For this review, take the finished solid that the model builds, in its own axes (mm). A direction names the side the tool comes from. Give positions to 0.01 mm unless a question says otherwise; leave off trailing zeros. Loops run counter-clockwise (first coordinate to the right, second up) from the corner with the lowest first, then second, coordinate; pieces in that order, holes last.
Autodesk Inventor part; units mm, degrees
ref_plane "YZ Plane" through (0, 0, 0) normal (1, 0, 0) x (0, 1, 0)
ref_plane "XZ Plane" through (0, 0, 0) normal (0, 1, 0) x (-1, 0, 0)
ref_plane "XY Plane" through (0, 0, 0) normal (0, 0, 1) x (1, 0, 0)
sketch "Boceto1" plane through (0, 0, 0) normal (1, 0, 0) x (0, 1, 0)
  line L0 (0, 0) -> (19, 0)
  line L1 (19, 0) -> (19, -90)
  line L2 (19, -90) -> (0, -90)
  line L3 (0, -90) -> (0, 0)
  line L4 (19, -7.5) -> (22, -7.5)
  line L5 (22, -7.5) -> (22, -22.5)
  line L6 (22, -22.5) -> (19, -22.5)
  line L7 (19, -22.5) -> (19, -7.5)
  line L8 (19, -27.5) -> (22, -27.5)
  line L9 (22, -27.5) -> (22, -42.5)
  line L10 (22, -42.5) -> (19, -42.5)
  line L11 (19, -42.5) -> (19, -27.5)
  line L12 (19, -47.5) -> (22, -47.5)
  line L13 (22, -47.5) -> (22, -62.5)
  line L14 (22, -62.5) -> (19, -62.5)
  line L15 (19, -62.5) -> (19, -47.5)
  line L16 (19, -67.5) -> (22, -67.5)
  line L17 (22, -67.5) -> (22, -82.5)
  line L18 (22, -82.5) -> (19, -82.5)
  line L19 (19, -82.5) -> (19, -67.5)
  line L20 (9.5, 0) -> (9.5, -90) construction
  line L21 (0, -7.5) -> (-3, -7.5)
  line L22 (-3, -7.5) -> (-3, -22.5)
  line L23 (-3, -22.5) -> (0, -22.5)
  line L24 (0, -22.5) -> (0, -7.5)
  line L25 (0, -27.5) -> (-3, -27.5)
  line L26 (-3, -27.5) -> (-3, -42.5)
  line L27 (-3, -42.5) -> (0, -42.5)
  line L28 (0, -42.5) -> (0, -27.5)
  line L29 (0, -47.5) -> (-3, -47.5)
  line L30 (-3, -47.5) -> (-3, -62.5)
  line L31 (-3, -62.5) -> (0, -62.5)
  line L32 (0, -62.5) -> (0, -47.5)
  line L33 (0, -67.5) -> (-3, -67.5)
  line L34 (-3, -67.5) -> (-3, -82.5)
  line L35 (-3, -82.5) -> (0, -82.5)
  line L36 (0, -82.5) -> (0, -67.5)
  point P0 (20.5, -7.5)
  point P1 (20.5, -27.5)
  point P2 (20.5, -47.5)
  point P3 (20.5, -67.5)
  point P4 (-1.5, -7.5)
  point P5 (-1.5, -27.5)
  point P6 (-1.5, -47.5)
  point P7 (-1.5, -67.5)
  point P8 (0, -22.5)
  point P9 (0, -27.5)
  point P10 (0, -42.5)
  point P11 (0, -47.5)
  point P12 (0, -62.5)
  point P13 (0, -67.5)
  point P14 (0, -82.5)
  point P15 (19, -82.5)
  point P16 (19, -67.5)
  point P17 (19, -62.5)
  point P18 (19, -47.5)
  point P19 (19, -42.5)
  point P20 (19, -27.5)
  point P21 (19, -22.5)
  point P22 (0, -7.5)
  dimension "d0" = 19
  dimension "d1" = 90
  dimension "d2" = 3
  dimension "d3" = 15
  dimension "d4" = 7.5
  dimension "d7" = 20
extrude "Extrusión1" add sketch "Boceto1" along normal blind 3
Item 1: The part is to be moulded in two halves that separate along Z. For faces 4 (the flat face through (1, 22, -15)), 5 (the flat face through (1, 20, -7.5)), 6 (the flat face through (1, 20, -47.5)), say which applies: released by +Z, released by -Z, zero draft, split by the parting line, or undercut.
Answer:
face 4: zero draft
face 5: released by +Z
face 6: undercut
Item 2: Take a section at A-A on z = -24. Give the boundary of the cut face in (x, y), and give its area (3 significant figures).
Answer:
outline: (0, 0) - (3, 0) - (3, 19) - (0, 19) - close
area: 57.0 mm2
Item 3: For L1, parallel to Z at x = 1, y = 20.75; L2, parallel to Y at x = 2.6, z = -47, list the stretches that pass through material, from the lowest coordinate up.
Answer:
L1: z = -82.5 to -67.5, -62.5 to -47.5, -42.5 to -27.5, -22.5 to -7.5
L2: y = 0 to 19
Item 4: Tool access review of faces 1 (the flat face through (1, -1, -47.5)), 2 (the flat face through (1, 19, -65)), 3 (the flat face through (1, 19, -86)): name each direction out of +Z, -Z, +X, -X, +Y, -Y from which nothing blocks a thin tool from reaching the whole face with its end or side.
Answer:
face 1: +X, -X, -Y
face 2: +X, -X, +Y
face 3: -Z, +X, -X, +Y
Item 5: Clearance check with flat-ended pins moving along their axes: pin 1 Ø1.5 at (x, y) = (2, 21) entering from +Z; pin 2 Ø1.5 at (x, y) = (1, -1.5) entering from -Z; pin 3 Ø0.9 at (x, z) = (1.5, -26) entering from +Y. State where each tip first meets the part, or that it passes through.
Answer:
pin 1: stops at z = -7.5
pin 2: stops at z = -82.5
pin 3: stops at y = 19
